```python
from build123d import *

# Parameters (mm, degrees)
ESBO_O1_R                = 5
RESSALTO_EXTRUS_O1_DEPTH = 6
ESBO_O2_R                = 4.25
RESSALTO_EXTRUS_O2_DEPTH = 8
ESBO_O3_W                = 0.5
ESBO_O3_H                = 3
RESSALTO_EXTRUS_O3_DEPTH = 6
ESBO_O4_W                = 1.442967266
ESBO_O4_H                = 2.423445024
CORTE_EXTRUS_O1_DEPTH    = 8.5
ESBO_O5_R                = 3.5
RESSALTO_EXTRUS_O4_DEPTH = 6.3
ESBO_O6_R                = 1.75
RESSALTO_EXTRUS_O5_DEPTH = 4
ESBO_O7_R                = 5
RESSALTO_EXTRUS_O6_DEPTH = 6.5


with BuildPart() as part:
    # Esboço1 → Ressalto-extrusão1 (new body)
    with BuildSketch(Plane(origin=(0, 0, 0), x_dir=(1, 0, 0), z_dir=(0, 1, 0))):
        Circle(ESBO_O1_R)
    extrude(amount=RESSALTO_EXTRUS_O1_DEPTH)

    # Esboço2 → Ressalto-extrusão2 (add)
    with BuildSketch(Plane.XZ):
        Circle(ESBO_O2_R)
    extrude(amount=RESSALTO_EXTRUS_O2_DEPTH)

    # Esboço3 → Ressalto-extrusão3 (add)
    with BuildSketch(Plane.XZ.offset(8)):
        with Locations((2.25, 0)):
            Rectangle(ESBO_O3_W, ESBO_O3_H)
        with Locations((-2.25, 0)):
            Rectangle(ESBO_O3_W, ESBO_O3_H)
    extrude(amount=RESSALTO_EXTRUS_O3_DEPTH)

    # Esboço4 → Corte-extrusão1 (cut, through all)
    with BuildSketch(Plane.ZY.offset(2.5)):
        with Locations((-0.007097641, -12.050464305)):
            Rectangle(ESBO_O4_W, ESBO_O4_H)
    extrude(amount=-CORTE_EXTRUS_O1_DEPTH, mode=Mode.SUBTRACT)

    # Esboço5 → Ressalto-extrusão4 (add)
    with BuildSketch(Plane(origin=(0, 6, 0), x_dir=(1, 0, 0), z_dir=(0, 1, 0))):
        Circle(ESBO_O5_R)
    extrude(amount=RESSALTO_EXTRUS_O4_DEPTH)

    # Esboço6 → Ressalto-extrusão5 (add)
    with BuildSketch(Plane(origin=(0, 12.3, 0), x_dir=(1, 0, 0), z_dir=(0, 1, 0))):
        Circle(ESBO_O6_R)
    extrude(amount=RESSALTO_EXTRUS_O5_DEPTH)

    # Esboço7 → Ressalto-extrusão6 (add)
    with BuildSketch(Plane(origin=(0, 16.3, 0), x_dir=(1, 0, 0), z_dir=(0, 1, 0))):
        Circle(ESBO_O7_R)
    extrude(amount=RESSALTO_EXTRUS_O6_DEPTH)


solid = part.part
```
Geometry check sheet. Reference: the model listing, model coordinates, mm. A direction names the side the tool comes from. Give positions to 0.01 mm unless a question says otherwise; leave off trailing zeros. Write each loop counter-clockwise with the first axis right and the second up, starting at its lowest first coordinate (ties: lowest second). Pieces come first, ordered by that corner, then holes. Notation, with made-up numbers: (68, 70) -> (78, 70) arc R3 cw to (78, 74) -> close; hole circle Ø6 at (24, 14.25). An arc over 180 degrees is marked (long way). One line per question, with ' | ' between items.
Item 1: Sectioned sample at C-C, the plane x = 0. Record the boundary of the cut face in (y, z).
Determined:
outline: (-8, -4.25) -> (0, -4.25) -> (0, -5) -> (6, -5) -> (6, -3.5) -> (12.3, -3.5) -> (12.3, -1.75) -> (16.3, -1.75) -> (16.3, -5) -> (22.8, -5) -> (22.8, 5) -> (16.3, 5) -> (16.3, 1.75) -> (12.3, 1.75) -> (12.3, 3.5) -> (6, 3.5) -> (6, 5) -> (0, 5) -> (0, 4.25) -> (-8, 4.25) -> close
Item 2: Sectioned sample at B-B, the plane x = -3. Record the boundary of the cut face in (y, z).
Determined:
outline: (-8, -3.01) -> (0, -3.01) -> (0, -4) -> (6, -4) -> (6, -1.8) -> (12.3, -1.8) -> (12.3, 1.8) -> (6, 1.8) -> (6, 4) -> (0, 4) -> (0, 3.01) -> (-8, 3.01) -> close; (16.3, -4) -> (22.8, -4) -> (22.8, 4) -> (16.3, 4) -> close
Item 3: Sectioned sample at A-A, the plane z = -2.25. Record the boundary of the cut face in (x, y).
Determined:
outline: (-4.47, 0) -> (-3.61, 0) -> (-3.61, -8) -> (3.61, -8) -> (3.61, 0) -> (4.47, 0) -> (4.47, 6) -> (2.68, 6) -> (2.68, 12.3) -> (-2.68, 12.3) -> (-2.68, 6) -> (-4.47, 6) -> close; (-4.47, 16.3) -> (4.47, 16.3) -> (4.47, 22.8) -> (-4.47, 22.8) -> close
Item 4: Access from +Z, -Z, +X, -X, +Y, -Y to the whole of each face (thin tool, end or side, straight path). Record for faces 5 (the flat face through (2.2, 6, 3.3)), 6 (the flat face through (2.5, -10, 0)), 7 (the flat face through (-2.5, -10, 0)), 8 (the cylindrical face through (2.285, -3.944, 3.584)), 9 (the flat face through (-2, -10, 0)).
Determined:
face 5: none | face 6: +Z, -Z, +X, -Y | face 7: +Z, -Z, -X, -Y | face 8: -Y | face 9: +Z, -Z, -Y
Item 5: Sectioned sample at D-D, the plane y = 5. Record the boundary of the cut face in (x, z), plus the area to 3 significant figures.
Determined:
outline: circle Ø10 at (0, 0) | area: 78.5 mm^2
Item 6: Draft check along Y on faces 1 (the flat face through (-2, 0, 4)), 2 (the flat face through (-2, 12.3, 1)), 3 (the flat face through (0, 22.8, 0)), 4 (the cylindrical face through (1.617, 14.272, 0.67)). Enter one of: released by +Y, released by -Y, zero draft, split by the parting line, or undercut.
Determined:
face 1: released by -Y | face 2: undercut | face 3: released by +Y | face 4: undercut
Item 7: Scan lines: line 1 along Y through (x, z) = (2.25, 0.25); line 2 along Y through (x, z) = (-4.5, 2); line 3 along X through (y, z) = (-11.5, -1). Record each from-to range of solid material in increasing order.
Determined:
line 1: -14 to -13.26, -10.84 to 12.3, 16.3 to 22.8 | line 2: 0 to 6, 16.3 to 22.8 | line 3: -2.5 to -2, 2 to 2.5
Item 8: Depth check by flat-ended pin: pin 1 (2.5 mm diameter, centred on y = -10, z = -0.5, fed in from -X); pin 2 (6 mm diameter, centred on x = 2.5, y = 14, fed in from -Z); pin 3 (4 mm diameter, centred on x = -4, y = 2.5, fed in from +Z); pin 4 (1 mm diameter, centred on y = 15.5, z = -3.5, fed in from +X). Enter the tip coordinate at first touch or a pass-through.
Determined:
pin 1: x = -2.5 | pin 2: z = -4.97 | pin 3: z = 4.58 | pin 4: through
